from build123d import *

# Parameters (mm, degrees)
BOSS_EXTRUDE1_DEPTH                  = 3.175
SKETCH2_R                            = 3.302
CUT_EXTRUDE1_DEPTH                   = 7.3500001
FILLET1_R                            = 2.54
SKETCH3_R                            = 1.27
CUT_EXTRUDE2_DEPTH                   = 7.3500001
F_3_64_0_04688_DIAMETER_HOLE4_D      = 1.190752
F_3_64_0_04688_DIAMETER_HOLE4_DEPTH  = 6.35
F_3_64_0_04688_DIAMETER_HOLE4_TIP    = 0.357737992
F_3_64_0_04688_DIAMETER_HOLE5_D      = 1.190752
F_3_64_0_04688_DIAMETER_HOLE5_DEPTH  = 6.35
F_3_64_0_04688_DIAMETER_HOLE5_TIP    = 0.357737992
F_3_64_0_04688_DIAMETER_HOLE8_D      = 1.190752
F_3_64_0_04688_DIAMETER_HOLE8_DEPTH  = 6.35
F_3_64_0_04688_DIAMETER_HOLE8_TIP    = 0.357737992
F_3_64_0_04688_DIAMETER_HOLE10_D     = 1.190752
F_3_64_0_04688_DIAMETER_HOLE10_DEPTH = 6.35
F_3_64_0_04688_DIAMETER_HOLE10_TIP   = 0.357737992
F_3_64_0_04688_DIAMETER_HOLE11_D     = 1.190752
F_3_64_0_04688_DIAMETER_HOLE11_DEPTH = 6.35
F_3_64_0_04688_DIAMETER_HOLE11_TIP   = 0.357737992
F_3_64_0_04688_DIAMETER_HOLE12_D     = 1.190752
F_3_64_0_04688_DIAMETER_HOLE12_DEPTH = 6.35
F_3_64_0_04688_DIAMETER_HOLE12_TIP   = 0.357737992
F_3_64_0_04688_DIAMETER_HOLE13_D     = 1.190752
F_3_64_0_04688_DIAMETER_HOLE13_DEPTH = 6.35
F_3_64_0_04688_DIAMETER_HOLE13_TIP   = 0.357737992
F_3_64_0_04688_DIAMETER_HOLE14_D     = 1.190752
F_3_64_0_04688_DIAMETER_HOLE14_DEPTH = 6.35
F_3_64_0_04688_DIAMETER_HOLE14_TIP   = 0.357737992


with BuildPart() as part:
    # Sketch1 → Boss-Extrude1 (new body, symmetric)
    with BuildSketch(Plane(origin=(0, 0, 0), x_dir=(0, 0, -1), z_dir=(1, 0, 0))):
        with BuildLine():
            ThreePointArc((-2.006494412, 28.159824422), (-0.039619207, 28.470921794), (1.948985172, 28.575))
            Line((1.948985172, 28.575), (15.875, 28.575))
            ThreePointArc((15.875, 28.575), (36.080576272, 20.205576272), (44.45, 0))
            Line((44.45, 0), (44.45, -6.190753211))
            ThreePointArc((44.45, -6.190753211), (37.893805907, -22.018805907), (22.065753211, -28.575))
            Line((22.065753211, -28.575), (8.382, -28.575))
            Line((8.382, -28.575), (8.382, -11.811))
            Line((8.382, -11.811), (-8.382, -11.811))
            Line((-8.382, -11.811), (-8.382, -28.575))
            Line((-8.382, -28.575), (-20.221173657, -28.575))
            ThreePointArc((-20.221173657, -28.575), (-28.345832171, -26.755566561), (-34.918545763, -21.644808297))
            add(Edge.make_bspline(
                [(-2.006494412, 28.159824422), (-30.496101023, 22.112541402), (-51.196498918, 9.980376605), (-41.193293746, -14.035586788), (-34.918545763, -21.644808297)],
                knots=[0.014282519, 0.014282519, 0.014282519, 0.014282519, 0.629767973, 0.915551688, 0.915551688, 0.915551688, 0.915551688], degree=3))
        make_face()
    extrude(amount=BOSS_EXTRUDE1_DEPTH, both=True)

    # Sketch2 → Cut-Extrude1 (cut, through all)
    with BuildSketch(Plane(origin=(3.175, 0, 0), x_dir=(0, 0, -1), z_dir=(1, 0, 0))):
        with Locations((8.911992586, 28.575)):
            Circle(SKETCH2_R)
    extrude(amount=-CUT_EXTRUDE1_DEPTH, mode=Mode.SUBTRACT)

    # Fillet1
    fillet1_edges = [part.edges().sort_by_distance(p)[0] for p in [
        (0, 28.575, -5.609992586),
        (0, 28.575, -12.213992586),
    ]]
    fillet(fillet1_edges, radius=FILLET1_R)

    # Sketch3 → Cut-Extrude2 (cut, through all)
    with BuildSketch(Plane(origin=(3.175, 0, 0), x_dir=(0, 0, -1), z_dir=(1, 0, 0))):
        with Locations((11.557, -8.636)):
            Circle(SKETCH3_R)
        with Locations((-11.557, -8.636)):
            Circle(SKETCH3_R)
    extrude(amount=-CUT_EXTRUDE2_DEPTH, mode=Mode.SUBTRACT)

    # 3/64 (0.04688) Diameter Hole4
    with Locations(Plane(origin=(0, 27.653661398, 4.33381955), x_dir=(0, -0.217552501, 0.97604862), z_dir=(0, 0.97604862, 0.217552501))):
        with Locations((0, 0)):
            Hole(F_3_64_0_04688_DIAMETER_HOLE4_D / 2, depth=F_3_64_0_04688_DIAMETER_HOLE4_DEPTH)
            with Locations((0, 0, -(F_3_64_0_04688_DIAMETER_HOLE4_DEPTH + F_3_64_0_04688_DIAMETER_HOLE4_TIP / 2))):  # 118° drill point
                Cone(0, F_3_64_0_04688_DIAMETER_HOLE4_D / 2, F_3_64_0_04688_DIAMETER_HOLE4_TIP, mode=Mode.SUBTRACT)

    # 3/64 (0.04688) Diameter Hole5
    with Locations(Plane(origin=(0, 28.575, 0), x_dir=(1, 0, 0), z_dir=(0, 1, 0))):
        with Locations((0, 14.807920641)):
            Hole(F_3_64_0_04688_DIAMETER_HOLE5_D / 2, depth=F_3_64_0_04688_DIAMETER_HOLE5_DEPTH)
            with Locations((0, 0, -(F_3_64_0_04688_DIAMETER_HOLE5_DEPTH + F_3_64_0_04688_DIAMETER_HOLE5_TIP / 2))):  # 118° drill point
                Cone(0, F_3_64_0_04688_DIAMETER_HOLE5_D / 2, F_3_64_0_04688_DIAMETER_HOLE5_TIP, mode=Mode.SUBTRACT)

    # 3/64 (0.04688) Diameter Hole8
    with Locations(Plane(origin=(0, 6.972553311, -43.58626351), x_dir=(0, -0.969773001, -0.244008865), z_dir=(0, 0.244008865, -0.969773001))):
        with Locations((0, 0)):
            Hole(F_3_64_0_04688_DIAMETER_HOLE8_D / 2, depth=F_3_64_0_04688_DIAMETER_HOLE8_DEPTH)
            with Locations((0, 0, -(F_3_64_0_04688_DIAMETER_HOLE8_DEPTH + F_3_64_0_04688_DIAMETER_HOLE8_TIP / 2))):  # 118° drill point
                Cone(0, F_3_64_0_04688_DIAMETER_HOLE8_D / 2, F_3_64_0_04688_DIAMETER_HOLE8_TIP, mode=Mode.SUBTRACT)

    # 3/64 (0.04688) Diameter Hole10
    with Locations(Plane(origin=(0, -20.468796932, -39.305009918), x_dir=(0, -0.770151297, 0.637861254), z_dir=(0, -0.637861254, -0.770151297))):
        with Locations((0, 0)):
            Hole(F_3_64_0_04688_DIAMETER_HOLE10_D / 2, depth=F_3_64_0_04688_DIAMETER_HOLE10_DEPTH)
            with Locations((0, 0, -(F_3_64_0_04688_DIAMETER_HOLE10_DEPTH + F_3_64_0_04688_DIAMETER_HOLE10_TIP / 2))):  # 118° drill point
                Cone(0, F_3_64_0_04688_DIAMETER_HOLE10_D / 2, F_3_64_0_04688_DIAMETER_HOLE10_TIP, mode=Mode.SUBTRACT)

    # 3/64 (0.04688) Diameter Hole11
    with Locations(Plane(origin=(0, -28.575, 0), x_dir=(-1, 0, 0), z_dir=(0, -1, 0))):
        with Locations((0, 10.922)):
            Hole(F_3_64_0_04688_DIAMETER_HOLE11_D / 2, depth=F_3_64_0_04688_DIAMETER_HOLE11_DEPTH)
            with Locations((0, 0, -(F_3_64_0_04688_DIAMETER_HOLE11_DEPTH + F_3_64_0_04688_DIAMETER_HOLE11_TIP / 2))):  # 118° drill point
                Cone(0, F_3_64_0_04688_DIAMETER_HOLE11_D / 2, F_3_64_0_04688_DIAMETER_HOLE11_TIP, mode=Mode.SUBTRACT)

    # 3/64 (0.04688) Diameter Hole12
    with Locations(Plane(origin=(0, 9.016155881, 42.122855847), x_dir=(0, 0.862463982, -0.506118444), z_dir=(0, 0.506118444, 0.862463982))):
        with Locations((0, 0)):
            Hole(F_3_64_0_04688_DIAMETER_HOLE12_D / 2, depth=F_3_64_0_04688_DIAMETER_HOLE12_DEPTH)
            with Locations((0, 0, -(F_3_64_0_04688_DIAMETER_HOLE12_DEPTH + F_3_64_0_04688_DIAMETER_HOLE12_TIP / 2))):  # 118° drill point
                Cone(0, F_3_64_0_04688_DIAMETER_HOLE12_D / 2, F_3_64_0_04688_DIAMETER_HOLE12_TIP, mode=Mode.SUBTRACT)

    # 3/64 (0.04688) Diameter Hole13
    with Locations(Plane(origin=(0, -25.802087057, 30.118594378), x_dir=(0, -0.519549644, -0.854440265), z_dir=(0, -0.854440265, 0.519549644))):
        with Locations((1e-09, 0)):
            Hole(F_3_64_0_04688_DIAMETER_HOLE13_D / 2, depth=F_3_64_0_04688_DIAMETER_HOLE13_DEPTH)
            with Locations((0, 0, -(F_3_64_0_04688_DIAMETER_HOLE13_DEPTH + F_3_64_0_04688_DIAMETER_HOLE13_TIP / 2))):  # 118° drill point
                Cone(0, F_3_64_0_04688_DIAMETER_HOLE13_D / 2, F_3_64_0_04688_DIAMETER_HOLE13_TIP, mode=Mode.SUBTRACT)

    # 3/64 (0.04688) Diameter Hole14
    with Locations(Plane(origin=(0, -28.575, 0), x_dir=(-1, 0, 0), z_dir=(0, -1, 0))):
        with Locations((0, -10.922)):
            Hole(F_3_64_0_04688_DIAMETER_HOLE14_D / 2, depth=F_3_64_0_04688_DIAMETER_HOLE14_DEPTH)
            with Locations((0, 0, -(F_3_64_0_04688_DIAMETER_HOLE14_DEPTH + F_3_64_0_04688_DIAMETER_HOLE14_TIP / 2))):  # 118° drill point
                Cone(0, F_3_64_0_04688_DIAMETER_HOLE14_D / 2, F_3_64_0_04688_DIAMETER_HOLE14_TIP, mode=Mode.SUBTRACT)


solid = part.part
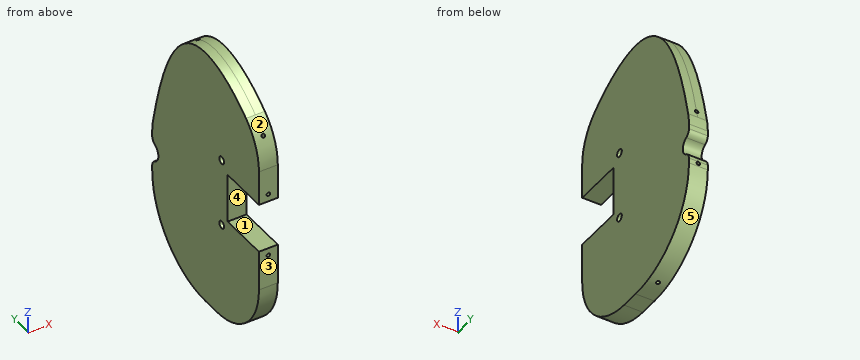
Part model, mm, in its own coordinate system. Face numbers are marked on the shaded views. A direction names the side the tool comes from. Coordinates: 2 decimals unless noted, no trailing zeros. Put each result on its own line as item: value.
1. Probe line 1 along Z through (x, y) = (2, -9); line 2 along Z through (x, y) = (-0.25, -7.5); line 3 along Z through (x, y) = (0, -24). List the from-to ranges inside material, lowest first. Write a range as [from, to].
Final values:
line 1: z = [-44.27, -12.77], [-10.34, 10.34], [12.77, 42.57]
line 2: z = [-44.41, -12.12], [-10.99, 10.99], [12.12, 43.11]
line 3: z = [-35.63, -11.52], [-10.33, -8.38], [8.38, 10.33], [11.52, 28.33], [29.72, 32.61]
2. Two-plate mould, pull along Z, no slides. Class the marked faces 3, 4 and 5: +Z half, -Z half, draft (parallel to the pull), parting line (faces both ways), or undercut.
Final values:
face 3: draft
face 4: undercut
face 5: -Z half
3. 3-axis set-ups, long thin cutter, end or side, ignore diameter. For the marked faces 1 and 2: which of +Z, -Z, +X, -X, +Y, -Y reach the whole face in a straight line?
Final values:
face 1: +X, -X, -Y
face 2: +Z, +X, -X, -Y
4. Band-saw the part on A-A (x = -1.5). Give the number of separate pieces and of enclosed holes in the cut face, then the cut area to 3 significant figures.
Final values:
separate pieces: 1
enclosed holes: 2
area: 3,990 mm²
5. Flat gauge pins, fed straight in: pin 1 Ø1.9 at (x, y) = (0, -23.5) entering from +Z; pin 2 Ø1.1 at (x, z) = (0, 10.922) entering from -Y; pin 3 Ø1.9 at (x, z) = (0.5, -1.5) entering from -Y; pin 4 Ø1.5 at (y, z) = (-8.636, -11.557) entering from +X. Where does each tip first touch, or does it go through?
Final values:
pin 1: stops at z = 34.12
pin 2: stops at y = -22.2
pin 3: stops at y = -11.81
pin 4: passes through
